Check sheet for the drawn part. Datum: minimum x, y, z corner. Units: mm. A direction names the side the tool comes from. Coordinates: 2 decimals unless noted, no trailing zeros. Loops run counter-clockwise (first coordinate to the right, second up) from the corner with the lowest first, then second, coordinate; pieces in that order, holes last.
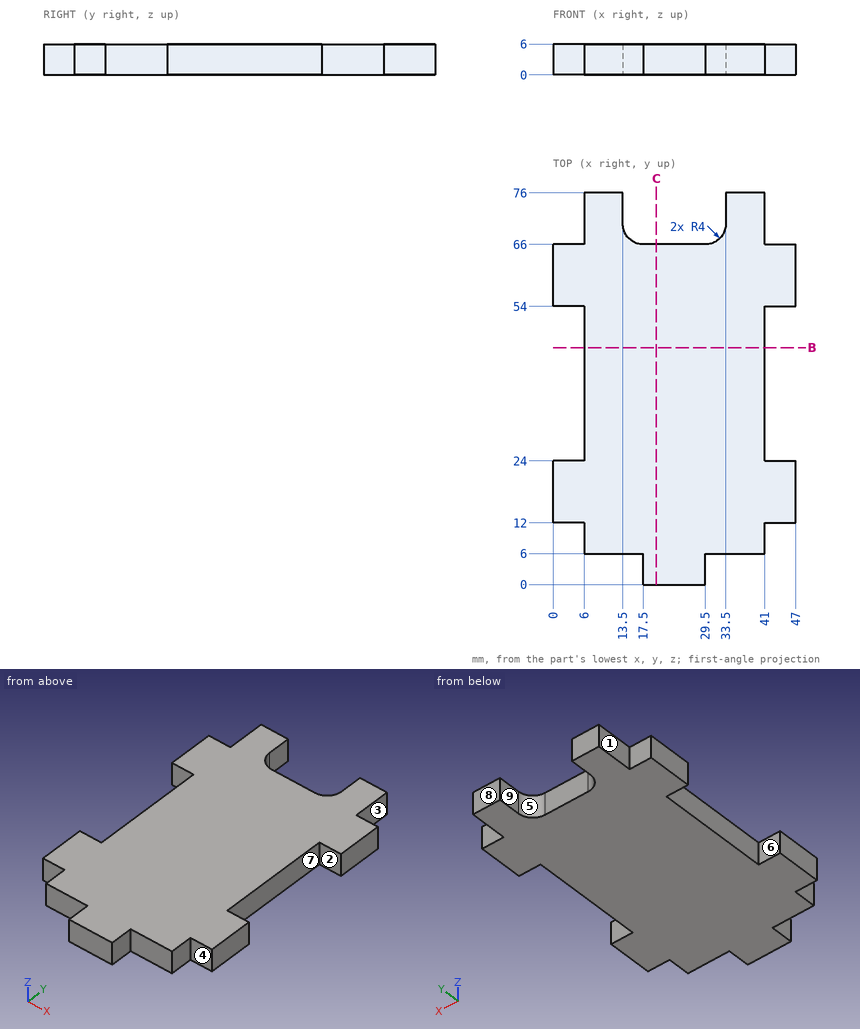
1) Set-up check for the marked faces 1, 2, 3, 4 and 5: record each of +Z, -Z, +X, -X, +Y, -Y from which the full face is reachable in a straight line by a thin tool's end or side.
Answer sheet:
face 1: +Z, -Z, -X, +Y
face 2: +Z, -Z, +X
face 3: +Z, -Z, +X, +Y
face 4: +Z, -Z, +X, -Y
face 5: +Z, -Z, +Y
2) Scan lines: line 1 (Y direction, x = 42, z = 4.05); line 2 (X direction, y = 27, z = 5.25); line 3 (Y direction, x = 24, z = 2.95). Record each from-to range of solid material in increasing order.
Answer sheet:
line 1: y = 12 to 24, 54 to 66
line 2: x = 6 to 41
line 3: y = 0 to 66
3) Section check C-C on x = 20. Enter the section's corners in (y, z), plus the area to 3 significant figures.
Answer sheet:
outline: (0, 0) - (66, 0) - (66, 6) - (0, 6) - close
area: 396 mm2
4) Mould release check, pull along Y, two halves, no side actions. Record for the marked faces 6, 7, 8 and 9: +Y half, -Y half, draft (parallel to the pull), parting line (faces both ways), or undercut.
Answer sheet:
face 6: undercut
face 7: undercut
face 8: +Y half
face 9: draft
5) Section check B-B on y = 46. Enter the section's corners in (x, z), plus the area to 3 significant figures.
Answer sheet:
outline: (6, 0) - (41, 0) - (41, 6) - (6, 6) - close
area: 210 mm2
6) Depth check by flat-ended pin: pin 1 (1.8 mm diameter, centred on x = 23, z = 3, fed in from +Y); pin 2 (3 mm diameter, centred on y = 70, z = 4.5, fed in from -X); pin 3 (3 mm diameter, centred on x = 2, z = 3.5, fed in from -Y). Enter the tip coordinate at first touch or a pass-through.
Answer sheet:
pin 1: stops at y = 66
pin 2: stops at x = 6
pin 3: stops at y = 12
